For this review, use the dimensioned drawing (mm, ordinates from the lowest corner) and the shaded views. A direction names the side the tool comes from. Coordinates: 2 decimals unless noted, no trailing zeros. Order: outer loops, then holes, each group sorted by start corner. A loop starts at its lowest first (then second) coordinate and runs counter-clockwise, first axis right, second up. Notation, with made-up numbers: M 51,38 L 107,38 A22 cw 107,51 Z; hole C -32,-24.5 d10. An arc over 180 degrees is marked long. Answer in a Markdown table with one row per item.
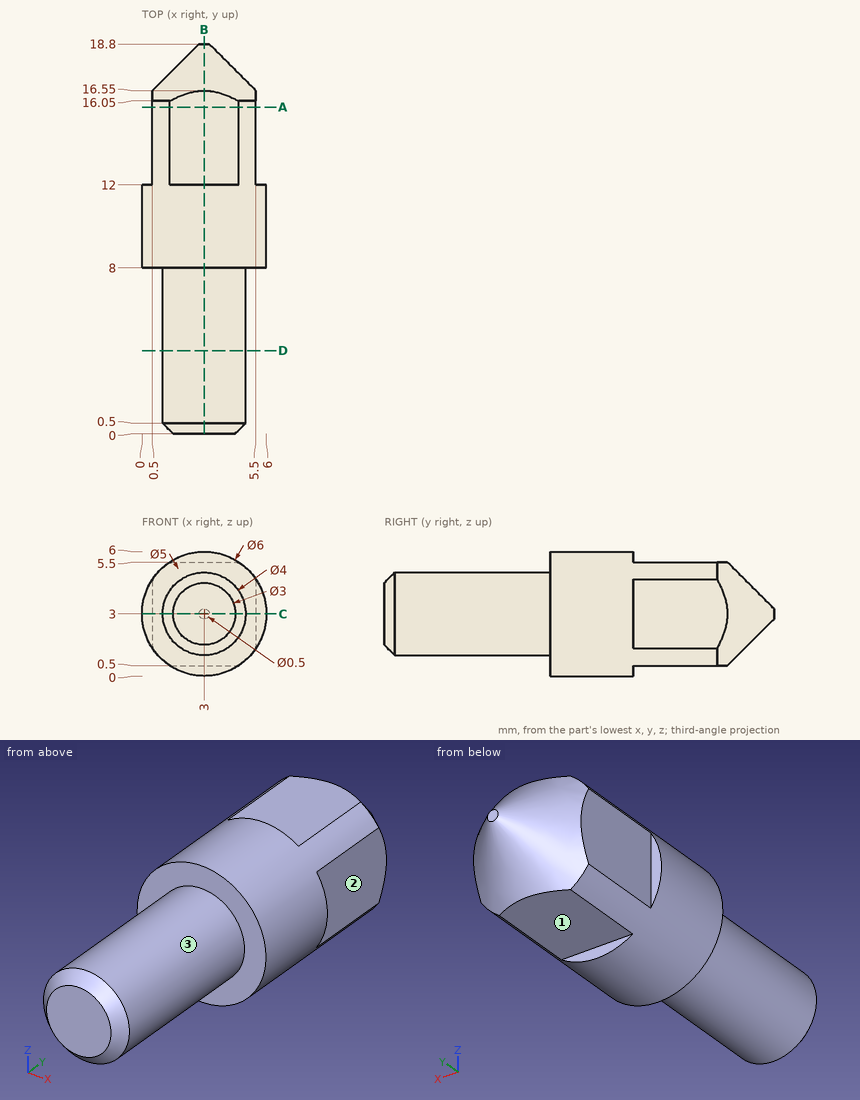
(1) Add section D-D, the plane y = 4. Give the boundary of the cut face in (x, z).
Return value:
| item | result |
|---|---|
| outline | C 3,3 d4 |
(2) For line 1 along Z through (x, y) = (4, 17.25); line 2 along Z through (x, y) = (2.3, 16); line 3 along X through (y, z) = (1.75, 3.65), list the stretches that pass through material, from the lowest coordinate up. Write a range as from..to.
Return value:
| item | result |
|---|---|
| line 1 | z = 1.5..4.5 |
| line 2 | z = 0.5..5.5 |
| line 3 | x = 1.11..4.89 |
(3) Insertion check: pin 1 Ø1.5 at (x, z) = (3, 2.5) entering from -Y; pin 2 Ø2.5 at (x, y) = (3, 14.5) entering from -Z; pin 3 Ø1 at (y, z) = (2.5, 1.5) entering from -X; pin 4 Ø3.5 at (y, z) = (14, 2.5) entering from +X. Each pin has a flat end and moves straight along its axis. Give the tip position at first contact, or say it passes through.
Return value:
| item | result |
|---|---|
| pin 1 | stops at y = 0 |
| pin 2 | stops at z = 0.5 |
| pin 3 | stops at x = 1.27 |
| pin 4 | stops at x = 5.5 |
(4) Add section C-C, the plane z = 3. Give the boundary of the cut face in (x, y).
Return value:
| item | result |
|---|---|
| outline | M 0,8 L 1,8 L 1,0.5 L 1.5,0 L 4.5,0 L 5,0.5 L 5,8 L 6,8 L 6,12 L 5.5,12 L 5.5,16.55 L 3.25,18.8 L 2.75,18.8 L 0.5,16.55 L 0.5,12 L 0,12 Z |
(5) For the marked faces 1, 2 and 3, list the 3-axis set-ups (+Z, -Z, +X, -X, +Y, -Y) from which the entire face can be reached by the end or side of a thin tool; tool diameter is ignored.
Return value:
| item | result |
|---|---|
| face 1 | -Z, +X, -X, +Y |
| face 2 | +Z, -Z, +X, +Y |
| face 3 | -Y |
(6) Add section B-B, the plane x = 3. Give the boundary of the cut face in (y, z).
Return value:
| item | result |
|---|---|
| outline | M 0,1.5 L 0.5,1 L 8,1 L 8,0 L 12,0 L 12,0.5 L 16.55,0.5 L 18.8,2.75 L 18.8,3.25 L 16.55,5.5 L 12,5.5 L 12,6 L 8,6 L 8,5 L 0.5,5 L 0,4.5 Z |
(7) Add section A-A, the plane y = 15.75. Give the boundary of the cut face in (x, z), and give its area (3 significant figures).
Return value:
| item | result |
|---|---|
| outline | M 0.5,1.34 A3 ccw 1.34,0.5 L 4.66,0.5 A3 ccw 5.5,1.34 L 5.5,4.66 A3 ccw 4.66,5.5 L 1.34,5.5 A3 ccw 0.5,4.66 Z |
| area | 23.8 mm2 |
